Check sheet for the modelled part. Datum: model origin and axes. Units: mm. A direction names the side the tool comes from. Round coordinates to 2 decimals unless told otherwise and drop trailing zeros. Loops run counter-clockwise (first coordinate to the right, second up) from the corner with the lowest first, then second, coordinate; pieces in that order, holes last. Notation, with made-up numbers: (5.25, 64.5) - (13.25, 64.5) arc R22 cw to (13.25, 88.5) - close; hole circle Ø4 at (-11, 55). An arc over 180 degrees is marked (long way). Return JSON: item names as keys, results as strings.
from build123d import *

# Parameters (mm, degrees)
F1_DEPTH = 63.5
F0_W     = 24.2118924779
F0_H     = 19.05
F2_DEPTH = 25.4
F3_DEPTH = 7.9375
F5_R     = 6.35


with BuildPart() as f1:
    # F0 (on Front) → F1 (new body, symmetric)
    with BuildSketch(Plane.XZ):
        Polygon((22.225, 9.525), (-41.275, 9.525), (-41.275, -9.525), (41.275, -9.525), (41.275, 9.525), align=None)
    extrude(amount=F1_DEPTH, both=True)

    # F0 (on Front) → F2 (join, symmetric)
    with BuildSketch(Plane.XZ):
        with BuildLine():
            Line((60.325, 42.8752), (60.325, 61.9252))
            Line((60.325, 61.9252), (57.15, 61.9252))
            ThreePointArc((57.15, 61.9252), (32.4542956671, 51.6959043329), (22.225, 27.0002))
            Line((22.225, 27.0002), (22.225, 9.525))
            Line((22.225, 9.525), (41.275, 9.525))
            Line((41.275, 9.525), (41.275, 27.0002))
            ThreePointArc((41.275, 27.0002), (45.9246798487, 38.2255201513), (57.15, 42.8752))
            Line((57.15, 42.8752), (60.325, 42.8752))
        make_face()
        with Locations((72.430946239, 52.4002)):
            Rectangle(F0_W, F0_H)
    extrude(amount=F2_DEPTH, both=True)

    # F0 (on Front) → F3 (join, symmetric)
    with BuildSketch(Plane.XZ):
        with BuildLine():
            ThreePointArc((22.225, 27.0002), (32.4542956671, 51.6959043329), (57.15, 61.9252))
            add(Edge.make_bspline(
                [(-41.275, 9.525), (-41.352327913, 28.8889557123), (19.8454335332, 62.4071657658), (57.15, 61.9252)],
                knots=[0, 0, 0, 0, 111.5045361635, 111.5045361635, 111.5045361635, 111.5045361635], degree=3))
            Line((-41.275, 9.525), (22.225, 9.525))
            Line((22.225, 9.525), (22.225, 27.0002))
        make_face()
    extrude(amount=F3_DEPTH, both=True)

    # F0 (on Front) → F4 (revolve)
    with BuildSketch(Plane.XZ):
        Polygon((111.125, 38.1), (111.125, 66.675), (84.5368924779, 66.675), (84.5368924779, 61.9252), (84.5368924779, 42.8752), (84.5368924779, 38.1), align=None)
    revolve(axis=Axis((84.5368924779, 0, 52.3875), (0, 0, 1)))

    # F5
    f5_edges = [f1.edges().sort_by_distance(p)[0] for p in [
        (-41.275, -63.5, 0),
        (41.275, -63.5, 0),
        (41.275, 63.5, 0),
        (-41.275, 63.5, 0),
    ]]
    fillet(f5_edges, radius=F5_R)


solid = f1.part
Q1. Scan lines: probe 1 along Z at (x, y) = (74.5, 1) (3 decimals); probe 2 along X at (y, z) = (-25.5, 3) (3 decimals); probe 3 along Z at (x, y) = (-14, 45) (3 decimals). Record each from-to range of solid material in increasing order. Write a range as [from, to].
Answer key:
{"probe 1": "z = [38.1, 66.675]", "probe 2": "x = [-41.275, 41.275]", "probe 3": "z = [-9.525, 9.525]"}
Q2. Sectioned sample at A-A (z = 3). Enter the section's corners in (x, y) (3 decimals).
Answer key:
{"outline": "(-41.275, -57.15) arc R6.35 ccw to (-34.925, -63.5) - (34.925, -63.5) arc R6.35 ccw to (41.275, -57.15) - (41.275, 57.15) arc R6.35 ccw to (34.925, 63.5) - (-34.925, 63.5) arc R6.35 ccw to (-41.275, 57.15) - close"}
Q3. Sectioned sample at B-B (y = -49.5). Enter the section's corners in (x, z) (3 decimals).
Answer key:
{"outline": "(-41.275, -9.525) - (41.275, -9.525) - (41.275, 9.525) - (-41.275, 9.525) - close"}
Q4. Sectioned sample at C-C (x = 97.5). Enter the section's corners in (y, z) (3 decimals).
Answer key:
{"outline": "(-23.214, 38.1) - (23.214, 38.1) - (23.214, 66.675) - (-23.214, 66.675) - close"}
Q5. Tool access check on faces 4 (the face through (22.225, 17, 18)), 5 (the face through (32.73, -16.79, 51.97)), 6 (the face through (57.6, -2, 61.925)), 7 (the face through (41.275, -1, 4)). Record the directions out of +Z, -Z, +X, -X, +Y, -Y that give a thin tool (end or side, any length) a straight path to the whole face; none if there is none.
Answer key:
{"face 4": "+Z, -X, +Y", "face 5": "+Z, -X, -Y", "face 6": "+Z, -X", "face 7": "-Z, +X, +Y, -Y"}
Q6. Depth check by flat-ended pin: P1, Ø6, axis at x = 65, y = 26.5, coming from the +Z side; P2, Ø4, axis at x = 73.5, z = 53.5, coming from the -Y side; P3, Ø11, axis at y = 22, z = 15, coming from the +X side (3 decimals); P4, Ø19, axis at y = 12.5, z = 14.5, coming from the -X side. Enter the tip coordinate at first touch or a pass-through.
Answer key:
{"P1": "stops at z = 61.93", "P2": "stops at y = -25.4", "P3": "stops at x = 41.275", "P4": "stops at x = -41.28"}
Q7. Sectioned sample at D-D (y = 20.5). Enter the section's corners in (x, z) (3 decimals), plus the area to 3 significant figures.
Answer key:
{"outline": "(-41.275, -9.525) - (41.275, -9.525) - (41.275, 27) arc R15.875 cw to (57.15, 42.875) - (67.605, 42.875) - (67.605, 38.1) - (101.468, 38.1) - (101.468, 66.675) - (67.605, 66.675) - (67.605, 61.925) - (57.15, 61.925) arc R34.925 ccw to (22.225, 27) - (22.225, 9.525) - (-41.275, 9.525) - close", "area": "3,830 mm²"}
Q8. Draft check along X on faces 1 (the face through (-41.275, -1, 0)), 2 (the face through (43, -25.4, 42)), 3 (the face through (45.8, -0.4, 38.1)). Enter one of: released by +X, released by -X, zero draft, split by the parting line, or undercut.
Answer key:
{"face 1": "released by -X", "face 2": "zero draft", "face 3": "undercut"}
